Input: part model. Units: mm. Frame: model coordinates. A direction names the side the tool comes from. Coordinates: 2 decimals unless noted, no trailing zeros. Put each result on its own line as item: value. Start each with the question number.
1. Pin query (flat end, axial travel): pin 1 (2 mm diameter, centred on x = 65, y = 0.5, fed in from +Z); pin 2 (2.5 mm diameter, centred on x = -66, y = 0, fed in from +Z). Return the tip coordinate at first contact, or that it passes through.
2. Pull-direction query (X, two-part tool) for faces 1 (the flat face through (-132, 0, 3)), 2 (the flat face through (-2, -11.5, 3)), 3 (the flat face through (66.7, 1.5, 2)); classes: released by +X, released by -X, zero draft, split by the parting line, or undercut.
3. Access query for faces 4 (the flat face through (-65.3, 1.5, 2)), 5 (the flat face through (132, 0, 3)). Directions: +Z, -Z, +X, -X, +Y, -Y. A direction counts if a zero-diameter tool reaches every point of the face in a straight line with its end or side. Return the directions, or none.
4. Line query: line 1 (X direction, y = 0, z = 0.85); line 2 (X direction, y = -1, z = 3.2); line 3 (Y direction, x = -66, z = 0.55). Output: solid intervals per line, ascending.
from build123d import *

# Parameters (mm, degrees)
SKETCH1_W           = 264
SKETCH1_H           = 23
SKETCH1_R           = 1.5
BOSS_EXTRUDE1_DEPTH = 5.8
SKETCH2_R           = 3.25
CUT_EXTRUDE1_DEPTH  = 3.8


with BuildPart() as part:
    # Sketch1 → Boss-Extrude1 (new body)
    with BuildSketch(Plane.XY):
        Rectangle(SKETCH1_W, SKETCH1_H)
        with Locations((-66, 0)):
            Circle(SKETCH1_R, mode=Mode.SUBTRACT)
        with Locations((66, 0)):
            Circle(SKETCH1_R, mode=Mode.SUBTRACT)
    extrude(amount=BOSS_EXTRUDE1_DEPTH)

    # Sketch2 → Cut-Extrude1 (cut)
    with BuildSketch(Plane.XY.offset(5.8)):
        with Locations((-66, 0)):
            Circle(SKETCH2_R)
        with Locations((66, 0)):
            Circle(SKETCH2_R)
    extrude(amount=-CUT_EXTRUDE1_DEPTH, mode=Mode.SUBTRACT)


solid = part.part
Report:
1. pin 1: stops at z = 2
1. pin 2: passes through
2. face 1: released by -X
2. face 2: zero draft
2. face 3: undercut
3. face 4: +Z
3. face 5: +Z, -Z, +X, +Y, -Y
4. line 1: x = -132 to -67.5, -64.5 to 64.5, 67.5 to 132
4. line 2: x = -132 to -69.09, -62.91 to 62.91, 69.09 to 132
4. line 3: y = -11.5 to -1.5, 1.5 to 11.5
